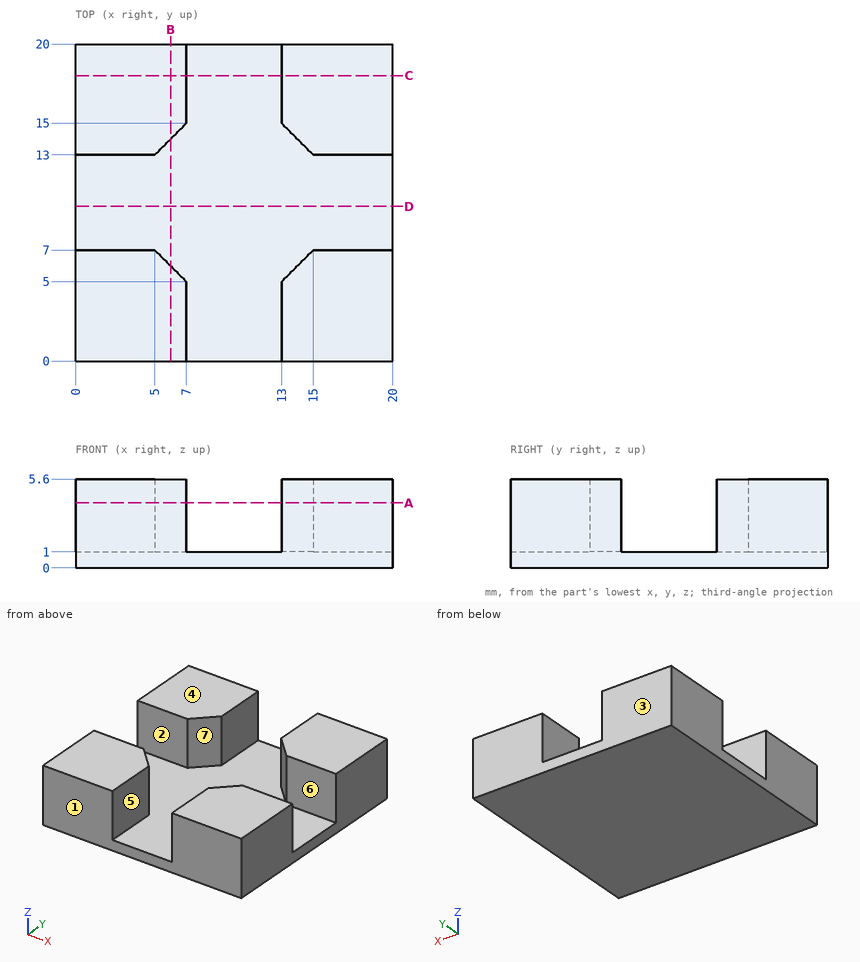
Source: three-view drawing plus pictorial views. Frame: mm from the lowest corner of the part. A direction names the side the tool comes from. Round coordinates to 2 decimals unless told otherwise and drop trailing zeros. Write each loop counter-clockwise with the first axis right and the second up, starting at its lowest first coordinate (ties: lowest second). Pieces come first, ordered by that corner, then holes. Notation, with made-up numbers: (33, 84) -> (45, 84) arc R24 ccw to (45, 98) -> close; hole circle Ø8 at (51, -16.5). An arc over 180 degrees is marked (long way). Return JSON: item names as keys, results as strings.
Q1. Section B-B on x = 6. Return the cut outline in (y, z), and give its area (3 significant figures).
From the geometry:
{"outline": "(0, 0) -> (20, 0) -> (20, 5.6) -> (14, 5.6) -> (14, 1) -> (6, 1) -> (6, 5.6) -> (0, 5.6) -> close", "area": "75.2 mm2"}
Q2. Set-up query: the marked faces 5, 6 and 7. Return all of +Z, -Z, +X, -X, +Y, -Y with unobstructed straight access to the full face (end or side cutting, diameter ignored); none if empty.
From the geometry:
{"face 5": "+Z, +Y, -Y", "face 6": "+Z, +X, -X", "face 7": "+Z"}
Q3. Ray query, line 1 (Y direction, x = 3, z = 2.7); line 2 (Z direction, x = 15.75, y = 11). Return the intervals inside material, ascending.
From the geometry:
{"line 1": "0 to 7, 13 to 20", "line 2": "0 to 1"}
Q4. Section D-D on y = 9.75. Return the cut outline in (x, z).
From the geometry:
{"outline": "(0, 0) -> (20, 0) -> (20, 1) -> (0, 1) -> close"}
Q5. Section A-A on z = 4.1. Return the cut outline in (x, y).
From the geometry:
{"outline": "(0, 0) -> (7, 0) -> (7, 5) -> (5, 7) -> (0, 7) -> close; (0, 13) -> (5, 13) -> (7, 15) -> (7, 20) -> (0, 20) -> close; (13, 0) -> (20, 0) -> (20, 7) -> (15, 7) -> (13, 5) -> close; (13, 15) -> (15, 13) -> (20, 13) -> (20, 20) -> (13, 20) -> close"}
Q6. Mould query, pull axis Y, two halves, no side actions, for the marked faces 1, 2, 3 and 4. Classes: +Y half, -Y half, draft (parallel to the pull), parting line (faces both ways), or undercut.
From the geometry:
{"face 1": "-Y half", "face 2": "undercut", "face 3": "+Y half", "face 4": "draft"}
Q7. Section C-C on y = 18. Return the cut outline in (x, z), and give its area (3 significant figures).
From the geometry:
{"outline": "(0, 0) -> (20, 0) -> (20, 5.6) -> (13, 5.6) -> (13, 1) -> (7, 1) -> (7, 5.6) -> (0, 5.6) -> close", "area": "84.4 mm2"}
